from build123d import *

# Parameters (mm, degrees)
SKETCH1_R           = 30.5
SKETCH1_R_2         = 25
BOSS_EXTRUDE1_DEPTH = 1.25
SKETCH2_R           = 30.5
BOSS_EXTRUDE2_DEPTH = 30
BOSS_EXTRUDE2_DRAFT = -60
SKETCH3_R           = 29.25
CUT_EXTRUDE1_DEPTH  = 30
CUT_EXTRUDE1_DRAFT  = 60
SKETCH4_R           = 94.674694241
SKETCH4_R_2         = 37
CUT_EXTRUDE2_DEPTH  = 30
SKETCH7_R           = 30.5
SKETCH7_R_2         = 25
BOSS_EXTRUDE4_DEPTH = 1.25
CUT_EXTRUDE3_DEPTH  = 30


with BuildPart() as part:
    # Sketch1 → Boss-Extrude1 (new body)
    with BuildSketch(Plane(origin=(0, 0, 0), x_dir=(1, 0, 0), z_dir=(0, 1, 0))):
        with Locations(Location((0, 0, 0), (0, 0, 270))):
            Circle(SKETCH1_R)
        with Locations(Location((0, 0, 0), (0, 0, 270))):
            Circle(SKETCH1_R_2, mode=Mode.SUBTRACT)
    extrude(amount=BOSS_EXTRUDE1_DEPTH)


with BuildPart() as boss_extrude2_tool:
    # Sketch2 → Boss-Extrude2 (with draft: the straight prism first)
    with BuildSketch(Plane(origin=(0, 0, 0), x_dir=(1, 0, 0), z_dir=(0, 1, 0))):
        Circle(SKETCH2_R)
    extrude(amount=BOSS_EXTRUDE2_DEPTH)
    # Boss-Extrude2: the draft: its side faces are tilted about the plane it starts from
    boss_extrude2_sides = [boss_extrude2_tool.faces().sort_by_distance(p)[0] for p in [
        (-30.5, 15, 0),
    ]]
    draft(boss_extrude2_sides, Plane(origin=(0, 0, 0), x_dir=(1, 0, 0), z_dir=(0, 1, 0)), BOSS_EXTRUDE2_DRAFT)


with BuildPart() as part_1:
    add(part.part)

    # Boss-Extrude2: add boss_extrude2_tool
    add(boss_extrude2_tool.part)


with BuildPart() as cut_extrude1_tool:
    # Sketch3 → Cut-Extrude1 (with draft: the straight prism first)
    with BuildSketch(Plane.XZ):
        Circle(SKETCH3_R)
    extrude(amount=-CUT_EXTRUDE1_DEPTH)
    # Cut-Extrude1: the draft: its side faces are tilted about the plane it starts from
    cut_extrude1_sides = [cut_extrude1_tool.faces().sort_by_distance(p)[0] for p in [
        (-29.25, 15, 0),
    ]]
    draft(cut_extrude1_sides, Plane.XZ, CUT_EXTRUDE1_DRAFT)


with BuildPart() as part_2:
    add(part_1.part)

    # Cut-Extrude1: cut by cut_extrude1_tool
    add(cut_extrude1_tool.part, mode=Mode.SUBTRACT)

    # Sketch4 → Cut-Extrude2 (cut)
    with BuildSketch(Plane(origin=(0, 0, 0), x_dir=(1, 0, 0), z_dir=(0, 1, 0))):
        Circle(SKETCH4_R)
        with Locations(Location((0, 0, 0), (0, 0, 270))):
            Circle(SKETCH4_R_2, mode=Mode.SUBTRACT)
    extrude(amount=CUT_EXTRUDE2_DEPTH, mode=Mode.SUBTRACT)

    # Sketch7 → Boss-Extrude4 (add)
    with BuildSketch(Plane(origin=(0, 0, 0), x_dir=(1, 0, 0), z_dir=(0, 1, 0))):
        with Locations(Location((0, 0, 0), (0, 0, 270))):
            Circle(SKETCH7_R)
        with Locations(Location((0, 0, 0), (0, 0, 270))):
            Circle(SKETCH7_R_2, mode=Mode.SUBTRACT)
    extrude(amount=BOSS_EXTRUDE4_DEPTH)

    # Sketch5 → Cut-Extrude3 (cut)
    with BuildSketch(Plane(origin=(0, 0, 0), x_dir=(1, 0, 0), z_dir=(0, 1, 0))):
        with BuildLine():
            Line((-36.878177829, 3), (-29.095747112, 3))
            ThreePointArc((-29.095747112, 3), (-28.751963166, 5.374673396), (-28.214701174, 7.713179477))
            Line((-28.214701174, 7.713179477), (-35.471601695, 10.524517717))
            ThreePointArc((-35.471601695, 10.524517717), (-36.370004688, 6.798732159), (-36.878177829, 3))
        make_face()
        with BuildLine():
            Line((-33.304151698, 16.119351093), (-26.047251177, 13.308012854))
            ThreePointArc((-26.047251177, 13.308012854), (-24.86885122, 15.398140764), (-23.5231035, 17.384651326))
            Line((-23.5231035, 17.384651326), (-29.274389198, 22.627640997))
            ThreePointArc((-29.274389198, 22.627640997), (-31.458034022, 19.477990026), (-33.304151698, 16.119351093))
        make_face()
        with BuildLine():
            Line((-25.232215336, 27.061694501), (-19.480929638, 21.81870483))
            ThreePointArc((-19.480929638, 21.81870483), (-17.627063114, 23.342003898), (-15.654580352, 24.708229682))
            Line((-15.654580352, 24.708229682), (-19.123508224, 31.674775977))
            ThreePointArc((-19.123508224, 31.674775977), (-22.297481546, 29.526637409), (-25.232215336, 27.061694501))
        make_face()
        with BuildLine():
            Line((-13.752528476, 34.349206112), (-10.283600604, 27.382659816))
            ThreePointArc((-10.283600604, 27.382659816), (-8.00464246, 28.133400063), (-5.671819382, 28.694824706))
            Line((-5.671819382, 28.694824706), (-6.389891497, 36.444056946))
            ThreePointArc((-6.389891497, 36.444056946), (-10.125530633, 35.587548797), (-13.752528476, 34.349206112))
        make_face()
        with BuildLine():
            Line((-0.415486439, 36.997667102), (0.302585676, 29.248434863))
            ThreePointArc((0.302585676, 29.248434863), (2.698849514, 29.125224657), (5.076952224, 28.80602465))
            Line((5.076952224, 28.80602465), (7.206715484, 36.29136608))
            ThreePointArc((7.206715484, 36.29136608), (3.4139293, 36.842164523), (-0.415486439, 36.997667102))
        make_face()
        with BuildLine():
            Line((12.977669343, 34.649388139), (10.847906083, 27.164046709))
            ThreePointArc((10.847906083, 27.164046709), (13.037846906, 26.183526272), (15.140053299, 25.026811345))
            Line((15.140053299, 25.026811345), (19.830015605, 31.237325128))
            ThreePointArc((19.830015605, 31.237325128), (16.492319164, 33.12104178), (12.977669343, 34.649388139))
        make_face()
        with BuildLine():
            Line((24.618118968, 27.621517309), (19.928156663, 21.411003527))
            ThreePointArc((19.928156663, 21.411003527), (21.616010829, 19.705597577), (23.158406283, 17.86758849))
            Line((23.158406283, 17.86758849), (29.775162236, 21.964510325))
            ThreePointArc((29.775162236, 21.964510325), (27.343329937, 24.926738815), (24.618118968, 27.621517309))
        make_face()
        with BuildLine():
            Line((32.933755213, 16.86320751), (26.31699926, 12.766285675))
            ThreePointArc((26.31699926, 12.766285675), (27.27481271, 10.566318736), (28.049088173, 8.295248801))
            Line((28.049088173, 8.295248801), (35.699008218, 9.725266693))
            ThreePointArc((35.699008218, 9.725266693), (34.501472488, 13.365941649), (32.933755213, 16.86320751))
        make_face()
        with BuildLine():
            ThreePointArc((29.25, 0), (29.225385963, -1.199714668), (29.15158528, -2.397410203))
            Line((29.15158528, -2.397410203), (36.801505325, -3.827428095))
            ThreePointArc((36.801505325, -3.827428095), (36.950343009, -1.916285858), (37, 0))
            ThreePointArc((37, 0), (36.950343009, 1.916285858), (36.801505325, 3.827428095))
            Line((36.801505325, 3.827428095), (29.15158528, 2.397410203))
            ThreePointArc((29.15158528, 2.397410203), (29.225385963, 1.199714668), (29.25, 0))
        make_face()
        with BuildLine():
            ThreePointArc((28.049088173, -8.295248801), (27.27481271, -10.566318736), (26.31699926, -12.766285675))
            Line((26.31699926, -12.766285675), (32.933755213, -16.86320751))
            ThreePointArc((32.933755213, -16.86320751), (34.501472488, -13.365941649), (35.699008218, -9.725266693))
            Line((35.699008218, -9.725266693), (28.049088173, -8.295248801))
        make_face()
        with BuildLine():
            ThreePointArc((23.158406283, -17.86758849), (21.616010829, -19.705597577), (19.928156663, -21.411003527))
            Line((19.928156663, -21.411003527), (24.618118968, -27.621517309))
            ThreePointArc((24.618118968, -27.621517309), (27.343329937, -24.926738815), (29.775162236, -21.964510325))
            Line((29.775162236, -21.964510325), (23.158406283, -17.86758849))
        make_face()
        with BuildLine():
            ThreePointArc((15.140053299, -25.026811345), (13.037846906, -26.183526272), (10.847906083, -27.164046709))
            Line((10.847906083, -27.164046709), (12.977669343, -34.649388139))
            ThreePointArc((12.977669343, -34.649388139), (16.492319164, -33.12104178), (19.830015605, -31.237325128))
            Line((19.830015605, -31.237325128), (15.140053299, -25.026811345))
        make_face()
        with BuildLine():
            ThreePointArc((5.076952224, -28.80602465), (2.698849514, -29.125224657), (0.302585676, -29.248434863))
            Line((0.302585676, -29.248434863), (-0.415486439, -36.997667102))
            ThreePointArc((-0.415486439, -36.997667102), (3.4139293, -36.842164523), (7.206715484, -36.29136608))
            Line((7.206715484, -36.29136608), (5.076952224, -28.80602465))
        make_face()
        with BuildLine():
            ThreePointArc((-5.671819382, -28.694824706), (-8.00464246, -28.133400063), (-10.283600604, -27.382659816))
            Line((-10.283600604, -27.382659816), (-13.752528476, -34.349206112))
            ThreePointArc((-13.752528476, -34.349206112), (-10.125530633, -35.587548797), (-6.389891497, -36.444056946))
            Line((-6.389891497, -36.444056946), (-5.671819382, -28.694824706))
        make_face()
        with BuildLine():
            ThreePointArc((-28.214701174, -7.713179477), (-28.751963166, -5.374673396), (-29.095747112, -3))
            Line((-29.095747112, -3), (-36.878177829, -3))
            ThreePointArc((-36.878177829, -3), (-36.370004688, -6.798732159), (-35.471601695, -10.524517717))
            Line((-35.471601695, -10.524517717), (-28.214701174, -7.713179477))
        make_face()
        with BuildLine():
            ThreePointArc((-23.5231035, -17.384651326), (-24.86885122, -15.398140764), (-26.047251177, -13.308012854))
            Line((-26.047251177, -13.308012854), (-33.304151698, -16.119351093))
            ThreePointArc((-33.304151698, -16.119351093), (-31.458034022, -19.477990026), (-29.274389198, -22.627640997))
            Line((-29.274389198, -22.627640997), (-23.5231035, -17.384651326))
        make_face()
        with BuildLine():
            ThreePointArc((-15.654580352, -24.708229682), (-17.627063114, -23.342003898), (-19.480929638, -21.81870483))
            Line((-19.480929638, -21.81870483), (-25.232215336, -27.061694501))
            ThreePointArc((-25.232215336, -27.061694501), (-22.297481546, -29.526637409), (-19.123508224, -31.674775977))
            Line((-19.123508224, -31.674775977), (-15.654580352, -24.708229682))
        make_face()
    extrude(amount=CUT_EXTRUDE3_DEPTH, mode=Mode.SUBTRACT)


solid = part_2.part
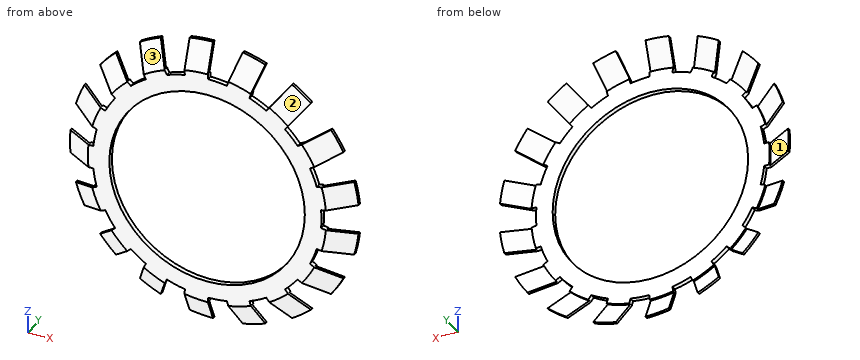
Input: part model. Units: mm. Frame: model coordinates. Face numbers are marked on the shaded views. Coordinates: 2 decimals unless noted, no trailing zeros. Write each question's results on one line, items separated by ' | '. Start each with the question number.
Q1. Ray query, line 1 (X direction, y = 1, z = 0); line 2 (Z direction, x = 2, y = 0.2); line 3 (Z direction, x = -26, y = 4.15). Return the intervals inside material, ascending. Write a range as from..to.
Q2. Section A-A, the plane x = -18. State how many separate pieces and enclosed holes the cut face has, plus the area to 3 significant figures.
Q3. Pin query (flat end, axial travel): pin 1 (1 mm diameter, centred on y = 1.5, z = -1.5, fed in from +X); pin 2 (1 mm diameter, centred on x = -22.5, y = 2.5, fed in from +Z); pin 3 (2 mm diameter, centred on x = 18.5, y = 1, fed in from +Z). Return the tip coordinate at first contact, or that it passes through.
Q4. Pull-direction query (X, two-part tool) for the marked faces 1, 2 and 3; classes: released by +X, released by -X, zero draft, split by the parting line, or undercut.
Found:
1) line 1: -32.23..-30.98, -30.5..-25, 25..29.25 | line 2: -29.18..-24.92, 24.92..29.18 | line 3: -26.32..-25.53, 25.53..26.32
2) separate pieces: 4 | enclosed holes: 0 | area: 18.5 mm2
3) pin 1: x = 29.23 | pin 2: z = 25.03 | pin 3: z = 28.58
4) face 1: undercut | face 2: released by +X | face 3: released by -X
